from build123d import *

# Parameters (mm, degrees)
F1_DEPTH      = 2438.4
F2_R          = 50.8
F3_DEPTH      = 55.5635
F4_R          = 50.8
F4_R_2        = 38.1
F5_DEPTH      = 46.0375
F5_DEPTH_BACK = 55.5625
F6_R          = 38.1
F7_DEPTH      = 1016
F7_DEPTH_BACK = 203.2


with BuildPart() as f1:
    # F0 (on Front) → F1 (new body)
    with BuildSketch(Plane.XZ):
        Polygon((-50.8, -101.6), (50.8, -101.6), (50.8, -95.25), (4.7625, -95.25), (4.7625, 95.25), (50.8, 95.25), (50.8, 101.6), (-50.8, 101.6), (-50.8, 95.25), (-4.7625, 95.25), (-4.7625, -95.25), (-50.8, -95.25), align=None)
    extrude(amount=-F1_DEPTH)

    # F2 (on face) → F3 (cut, through all)
    with BuildSketch(Plane.YZ.offset(4.7625)):
        with Locations((1168.4, 0)):
            Circle(F2_R)
        with Locations((1930.4, 0)):
            Circle(F2_R)
    extrude(amount=-F3_DEPTH, mode=Mode.SUBTRACT)

    # F4 (on face) → F5 (join, two sides)
    with BuildSketch(Plane.YZ.offset(4.7625)) as f5_sk:
        with Locations((1168.4, 0)):
            Circle(F4_R)
        with Locations((1168.4, 0)):
            Circle(F4_R_2, mode=Mode.SUBTRACT)
        with Locations((1930.4, 0)):
            Circle(F4_R)
        with Locations((1930.4, 0)):
            Circle(F4_R_2, mode=Mode.SUBTRACT)
    extrude(amount=F5_DEPTH)
    extrude(f5_sk.sketch, amount=-F5_DEPTH_BACK)

    # F6 (on face) → F7 (join, two sides)
    with BuildSketch(Plane.YZ.offset(50.8)) as f7_sk:
        with Locations((1168.4, 0)):
            Circle(F6_R)
        with Locations((1930.4, 0)):
            Circle(F6_R)
    extrude(amount=F7_DEPTH)
    extrude(f7_sk.sketch, amount=-F7_DEPTH_BACK)


solid = f1.part
Part model, mm, in its own coordinate system. A direction names the side the tool comes from. Coordinates: 2 decimals unless noted, no trailing zeros. Write each loop counter-clockwise with the first axis right and the second up, starting at its lowest first coordinate (ties: lowest second). Pieces come first, ordered by that corner, then holes. Notation, with made-up numbers: M -34,5 L 10,5 A13 ccw 10,25 Z; hole C 31.5,43 d8. An arc over 180 degrees is marked long. Return JSON: item names as keys, results as strings.
1. Probe L1, parallel to Y at x = 450.5, z = -0.5; L2, parallel to X at y = 1180, z = 71; L3, parallel to Y at x = 559, z = 17. List the from-to ranges inside material, lowest first.
Determined:
{"L1": "1130.3 to 1206.5, 1892.3 to 1968.5", "L2": "-4.76 to 4.76", "L3": "1134.3 to 1202.5, 1896.3 to 1964.5"}
2. Saw through at B-B, the plane x = 940. Write the cut outline in (y, z).
Determined:
{"outline": "C 1168.4,0 d76.2; C 1930.4,0 d76.2"}
3. 3-axis set-ups, long thin cutter, end or side, ignore diameter. For faces 1 (the face through (-27, 1202, -95.25)), 2 (the face through (551.69, 1966.74, 11.44)), 3 (the face through (-4.762, 1202, -41)), 4 (the face through (28, 1202, -95.25)), 5 (the face through (-152.4, 1168, 1)): which of +Z, -Z, +X, -X, +Y, -Y reach the whole face in a straight line?
Determined:
{"face 1": "-X, +Y, -Y", "face 2": "+X", "face 3": "-X", "face 4": "+X, +Y, -Y", "face 5": "+Z, -Z, -X, +Y, -Y"}
4. Flat gauge pins, fed straight in: pin 1 Ø2 at (x, z) = (302.5, 18.5) entering from -Y; pin 2 Ø5 at (y, z) = (684, 99) entering from +X; pin 3 Ø12 at (x, z) = (652, -2.5) entering from +Y. Where does each tip first touch, or does it go through?
Determined:
{"pin 1": "y = 1134.56", "pin 2": "x = 50.8", "pin 3": "y = 1968.5"}
5. Saw through at C-C, the plane y = 1930.4. Write the cut outline in (x, z), then the cut area to 3 significant figures.
Determined:
{"outline": "M -152.4,-38.1 L -50.8,-38.1 L -50.8,-50.8 L -4.76,-50.8 L -4.76,-95.25 L -50.8,-95.25 L -50.8,-101.6 L 50.8,-101.6 L 50.8,-95.25 L 4.76,-95.25 L 4.76,-50.8 L 50.8,-50.8 L 50.8,-38.1 L 1066.8,-38.1 L 1066.8,38.1 L 50.8,38.1 L 50.8,50.8 L 4.76,50.8 L 4.76,95.25 L 50.8,95.25 L 50.8,101.6 L -50.8,101.6 L -50.8,95.25 L -4.76,95.25 L -4.76,50.8 L -50.8,50.8 L -50.8,38.1 L -152.4,38.1 Z", "area": "97,600 mm²"}
6. Saw through at A-A, the plane y = 319.5. Write the cut outline in (x, z), then the cut area to 3 significant figures.
Determined:
{"outline": "M -50.8,-101.6 L 50.8,-101.6 L 50.8,-95.25 L 4.76,-95.25 L 4.76,95.25 L 50.8,95.25 L 50.8,101.6 L -50.8,101.6 L -50.8,95.25 L -4.76,95.25 L -4.76,-95.25 L -50.8,-95.25 Z", "area": "3,100 mm²"}
7. Pull direction Y, two halves, no side cores. Call faces 6 (the face through (-50.8, 1938, 38)), 7 (the face through (27, 1202, 95.25)), 8 (the face through (0, 0, 0)): pulls with the +Y half, pulls with the -Y half, needs draft (parallel to the pull), parting line crosses it, or undercut.
Determined:
{"face 6": "undercut", "face 7": "needs draft", "face 8": "pulls with the -Y half"}
